The model under review builds one solid part; all positions refer to its coordinate system, in mm. A direction names the side the tool comes from. Give positions to 0.01 mm unless a question says otherwise; leave off trailing zeros. Write each loop counter-clockwise with the first axis right and the second up, starting at its lowest first coordinate (ties: lowest second). Pieces come first, ordered by that corner, then holes. Notation, with made-up numbers: (-36, 30) -> (-25, 30) arc R17 ccw to (-25, 49) -> close; hole circle Ø4 at (65.5, 88.25). An arc over 180 degrees is marked (long way). Use CSV: the item, a comma, the result in double quotes.
```python
from build123d import *

# Parameters (mm, degrees)
BOSS_EXTRUDE1_DEPTH                     = 25.4
CBORE_FOR_M5_HEX_HEAD_BOLT1_D           = 3.5
CBORE_FOR_M5_HEX_HEAD_BOLT1_CBORE_D     = 6
CBORE_FOR_M5_HEX_HEAD_BOLT1_CBORE_DEPTH = 10
CHAMFER2_SIZE                           = 1.5
SKETCH7_R                               = 2.25
CUT_EXTRUDE1_DEPTH                      = 6.35
BOSS_EXTRUDE2_START                     = -0.12
SKETCH8_R                               = 1.75
BOSS_EXTRUDE2_DEPTH                     = 0.12


with BuildPart() as part:
    # Sketch1 → Boss-Extrude1 (new body)
    with BuildSketch(Plane.XY):
        Polygon((0, 0), (0, -15.24), (-48.05, -15.24), (-48.05, -21.59), (6.35, -21.59), (19.29, 0), (6.35, 0), align=None)
    extrude(amount=BOSS_EXTRUDE1_DEPTH)

    # CBORE for M5 Hex Head Bolt1 (through all)
    with Locations(Plane(origin=(5, -21.59, 20.2), x_dir=(-1, 0, 0), z_dir=(0, -1, 0))):
        with Locations((0, 0), (0, 7.5), (0, 15)):
            CounterBoreHole(CBORE_FOR_M5_HEX_HEAD_BOLT1_D / 2, CBORE_FOR_M5_HEX_HEAD_BOLT1_CBORE_D / 2, CBORE_FOR_M5_HEX_HEAD_BOLT1_CBORE_DEPTH)

    # Chamfer2
    chamfer2_edges = [part.edges().sort_by_distance(p)[0] for p in [
        (-48.05, -15.24, 12.7),
        (0, -15.24, 12.7),
        (-20.85, -21.59, 25.4),
        (12.82, -10.795, 25.4),
        (12.82, -10.795, 0),
        (-20.85, -21.59, 0),
    ]]
    chamfer(chamfer2_edges, length=CHAMFER2_SIZE)

    # Sketch7 → Cut-Extrude1 (cut)
    with BuildSketch(Plane.XZ.offset(21.59)):
        with Locations(Location((-29, 12.7, 0), (0, 0, 270))):
            Circle(SKETCH7_R)
    extrude(amount=-CUT_EXTRUDE1_DEPTH, mode=Mode.SUBTRACT)

    # Sketch8 → Boss-Extrude2 (add)
    with BuildSketch(Plane.XZ.offset(11.59).offset(BOSS_EXTRUDE2_START)):
        with Locations(Location((5, 20.2, 0), (0, 0, 270))):
            Circle(SKETCH8_R)
        with Locations(Location((5, 12.7, 0), (0, 0, 270))):
            Circle(SKETCH8_R)
        with Locations(Location((5, 5.2, 0), (0, 0, 270))):
            Circle(SKETCH8_R)
    extrude(amount=BOSS_EXTRUDE2_DEPTH)


solid = part.part
```
Q1. Consider section B-B (y = -16). Write out the cut boundary in (x, z), then the cut area to 3 significant figures.
Derived:
outline,"(-47.31, 0) -> (7.95, 0) -> (9.7, 1.5) -> (9.7, 23.9) -> (7.95, 25.4) -> (-47.31, 25.4) -> close; hole circle Ø4.5 at (-29, 12.7); hole circle Ø6 at (5, 5.2); hole circle Ø6 at (5, 12.7); hole circle Ø6 at (5, 20.2)"
area,"1,340 mm2"
Q2. Consider section A-A (x = -29). Write out the cut boundary in (y, z).
Derived:
outline,"(-21.59, 1.5) -> (-20.09, 0) -> (-15.24, 0) -> (-15.24, 10.45) -> (-21.59, 10.45) -> close; (-21.59, 14.95) -> (-15.24, 14.95) -> (-15.24, 25.4) -> (-20.09, 25.4) -> (-21.59, 23.9) -> close"
Q3. Consider section D-D (y = -3.25). Write out the cut boundary in (x, z).
Derived:
outline,"(0, 0) -> (15.59, 0) -> (17.34, 1.5) -> (17.34, 23.9) -> (15.59, 25.4) -> (0, 25.4) -> close; hole circle Ø3.5 at (5, 5.2); hole circle Ø3.5 at (5, 12.7); hole circle Ø3.5 at (5, 20.2)"
Q4. Machinability: for faces 4 (the flat face through (0, -7, 13)), 5 (the cylindrical face through (5.9, -5.7, 3.7)), 6 (the cylindrical face through (2.14, -16.66, 11.8)), which of the approach directions +Z, -Z, +X, -X, +Y, -Y give a long, thin tool a straight path to every point of the face, cutting with its end or side? Answer none if there is none.
Derived:
face 4,"+Z, -Z, -X, +Y"
face 5,"+Y"
face 6,"-Y"
Q5. Consider section C-C (z = 13.75). Write out the cut boundary in (x, y).
Derived:
outline,"(-48.05, -21.59) -> (-30.99, -21.59) -> (-30.99, -15.24) -> (-46.55, -15.24) -> (-48.05, -16.74) -> close; (-27.01, -21.59) -> (2.19, -21.59) -> (2.19, -11.59) -> (7.81, -11.59) -> (7.81, -19.15) -> (19.29, 0) -> (6.4, 0) -> (6.4, -11.47) -> (3.6, -11.47) -> (3.6, 0) -> (0, 0) -> (0, -13.74) -> (-1.5, -15.24) -> (-27.01, -15.24) -> close"
Q6. The part is to be moulded in two halves that separate along X. For faces 1 (the flat face through (-47.31, -16, 12.52)), 2 (the flat face through (-21.23, -20.85, 0.76)), 3 (the cylindrical face through (4.772, -5.655, 18.465)), say which applies: pulls with the +X half, pulls with the -X half, needs draft (parallel to the pull), parting line crosses it, or undercut.
Derived:
face 1,"pulls with the -X half"
face 2,"needs draft"
face 3,"undercut"
Q7. To check wall thickness, follow probe 1 along Z at (x, y) = (5, -17.25); probe 2 along Z at (x, y) = (5, -7); probe 3 along X at (y, z) = (-18.5, 20.2). State the ranges of each line that lie inside material, in increasing order.
Derived:
probe 1,"z = 0 to 2.2, 8.2 to 9.7, 15.7 to 17.2, 23.2 to 25.4"
probe 2,"z = 0 to 3.45, 6.95 to 10.95, 14.45 to 18.45, 21.95 to 25.4"
probe 3,"x = -48.05 to 2, 8 to 8.2"
Q8. Insertion check: pin 1 (5.5 mm diameter, centred on x = 5, z = 12.7, fed in from -Y); pin 2 (8 mm diameter, centred on y = -9.5, z = 5.5, fed in from -X); pin 3 (3 mm diameter, centred on y = -19, z = 13, fed in from +X). Each pin has a flat end and moves straight along its axis. Give the tip position at first contact, or say it passes through.
Derived:
pin 1,"stops at y = -11.59"
pin 2,"stops at x = 0"
pin 3,"stops at x = 8.8"
